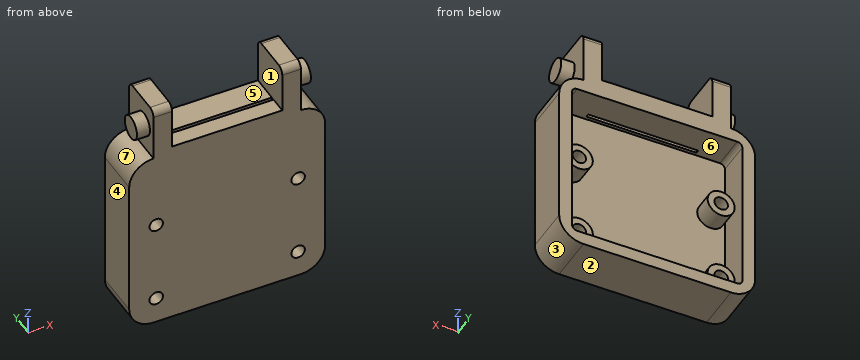
```python
from build123d import *

# Parameters (mm, degrees)
BOSS_EXTRUDE1_DEPTH   = 7
SKETCH2_R             = 2
CUT_EXTRUDE2_DEPTH    = 5
SKETCH3_R             = 2
CUT_EXTRUDE3_DEPTH    = 2
SKETCH4_W             = 16.3
SKETCH4_H             = 0.5
CUT_EXTRUDE4_DEPTH    = 2
F_2_0MM_DOWEL_HOLE1_D = 2
SKETCH8_W             = 21.826362025
SKETCH8_H             = 7
SKETCH8_W_2           = 16.3
SKETCH8_H_2           = 0.5
BOSS_EXTRUDE2_DEPTH   = 8
SKETCH9_R             = 1.75
BOSS_EXTRUDE3_DEPTH   = 2
LPATTERN4_COUNT       = 2
LPATTERN4_PITCH       = 23.75
SKETCH10_W            = 16.3
SKETCH10_H            = 7
CUT_EXTRUDE5_DEPTH    = 7
FILLET1_R             = 1


with BuildPart() as part:
    # Sketch1 → Boss-Extrude1 (new body)
    with BuildSketch(Plane(origin=(0, 0, 0), x_dir=(1, 0, 0), z_dir=(0, 1, 0))):
        with BuildLine():
            Line((-12.921525848, 14.392842997), (-12.921525848, -6.433519028))
            ThreePointArc((-12.921525848, -6.433519028), (-11.87097089, -8.969783057), (-9.334706861, -10.020338016))
            Line((-9.334706861, -10.020338016), (12.491655164, -10.020338016))
            ThreePointArc((12.491655164, -10.020338016), (15.027919193, -8.969783057), (16.078474152, -6.433519028))
            Line((16.078474152, -6.433519028), (16.078474152, 14.392842997))
            ThreePointArc((16.078474152, 14.392842997), (15.027919193, 16.929107026), (12.491655164, 17.979661984))
            Line((12.491655164, 17.979661984), (-9.334706861, 17.979661984))
            ThreePointArc((-9.334706861, 17.979661984), (-11.87097089, 16.929107026), (-12.921525848, 14.392842997))
        make_face()
    extrude(amount=BOSS_EXTRUDE1_DEPTH)

    # Sketch2 → Cut-Extrude2 (cut)
    with BuildSketch(Plane(origin=(0, 7, 0), x_dir=(1, 0, 0), z_dir=(0, 1, 0))):
        with BuildLine():
            Line((-10.27448552, 16.079661984), (13.431433823, 16.079661984))
            ThreePointArc((13.431433823, 16.079661984), (13.959671105, 15.860858938), (14.178474152, 15.332621656))
            Line((14.178474152, 15.332621656), (14.178474152, -7.373297687))
            ThreePointArc((14.178474152, -7.373297687), (13.959671105, -7.901534969), (13.431433823, -8.120338016))
            Line((13.431433823, -8.120338016), (-10.27448552, -8.120338016))
            ThreePointArc((-10.27448552, -8.120338016), (-10.802722802, -7.901534969), (-11.021525848, -7.373297687))
            Line((-11.021525848, -7.373297687), (-11.021525848, 15.332621656))
            ThreePointArc((-11.021525848, 15.332621656), (-10.802722802, 15.860858938), (-10.27448552, 16.079661984))
        make_face()
        with Locations((-8.921525848, 13.979661984)):
            Circle(SKETCH2_R, mode=Mode.SUBTRACT)
        with Locations((12.078474152, 13.979661984)):
            Circle(SKETCH2_R, mode=Mode.SUBTRACT)
        with Locations((-8.921525848, 1.479661984)):
            Circle(SKETCH2_R, mode=Mode.SUBTRACT)
        with Locations((12.078474152, 1.479661984)):
            Circle(SKETCH2_R, mode=Mode.SUBTRACT)
    extrude(amount=-CUT_EXTRUDE2_DEPTH, mode=Mode.SUBTRACT)

    # Sketch3 → Cut-Extrude3 (cut)
    with BuildSketch(Plane(origin=(0, 7, 0), x_dir=(1, 0, 0), z_dir=(0, 1, 0))):
        with Locations((12.078474152, 13.979661984)):
            Circle(SKETCH3_R)
        with Locations((12.078474152, 1.479661984)):
            Circle(SKETCH3_R)
        with Locations((-8.921525848, 13.979661984)):
            Circle(SKETCH3_R)
        with Locations((-8.921525848, 1.479661984)):
            Circle(SKETCH3_R)
    extrude(amount=-CUT_EXTRUDE3_DEPTH, mode=Mode.SUBTRACT)

    # Sketch4 → Cut-Extrude4 (cut)
    with BuildSketch(Plane.XY.offset(10.020338016)):
        with Locations((1.578474152, 2.75)):
            Rectangle(SKETCH4_W, SKETCH4_H)
    extrude(amount=-CUT_EXTRUDE4_DEPTH, mode=Mode.SUBTRACT)

    # Ø2.0mm Dowel Hole1 (through all)
    with Locations(Plane(origin=(0, 5, 0), x_dir=(1, 0, 0), z_dir=(0, 1, 0))):
        with Locations((12.078474152, 1.479661984), (12.078474152, 13.979661984), (-8.921525848, 1.479661984), (-8.921525848, 13.979661984)):
            Hole(F_2_0MM_DOWEL_HOLE1_D / 2)

    # Sketch8 → Boss-Extrude2 (add)
    with BuildSketch(Plane.XY.offset(10.020338016)):
        with Locations((1.578474152, 3.5)):
            Rectangle(SKETCH8_W, SKETCH8_H)
        with Locations((1.578474152, 2.75)):
            Rectangle(SKETCH8_W_2, SKETCH8_H_2, mode=Mode.SUBTRACT)
    extrude(amount=BOSS_EXTRUDE2_DEPTH)

    # Sketch9 → Boss-Extrude3 (add)
    with BuildSketch(Plane(origin=(12.491655164, 0, 0), x_dir=(0, 0, -1), z_dir=(1, 0, 0))):
        with Locations((-14.020338016, 2.75)):
            Circle(SKETCH9_R)
    boss_extrude3 = extrude(amount=BOSS_EXTRUDE3_DEPTH)

    # LPattern4: Boss-Extrude3 ×2
    with Locations(*[(-i * LPATTERN4_PITCH, 0, 0) for i in range(1, LPATTERN4_COUNT)]):
        add(boss_extrude3)

    # Sketch10 → Cut-Extrude5 (cut)
    with BuildSketch(Plane.XY.offset(18.020338016)):
        with Locations((1.578474152, 3.5)):
            Rectangle(SKETCH10_W, SKETCH10_H)
    extrude(amount=-CUT_EXTRUDE5_DEPTH, mode=Mode.SUBTRACT)

    # Fillet1
    fillet1_edges = [part.edges().sort_by_distance(p)[0] for p in [
        (-7.953116354, 0, 18.020338016),
        (11.110064658, 7, 18.020338016),
        (11.110064658, 0, 18.020338016),
        (-7.953116354, 7, 18.020338016),
    ]]
    fillet(fillet1_edges, radius=FILLET1_R)


solid = part.part
```
The listing builds one solid part. Answer for the finished solid, in the listing's coordinates (mm). Face numbers are marked on the shaded views. A direction names the side the tool comes from. Coordinates: 2 decimals unless noted, no trailing zeros. Loops run counter-clockwise (first coordinate to the right, second up) from the corner with the lowest first, then second, coordinate; pieces in that order, holes last. Notation, with made-up numbers: M 47.5,89 L 75.5,89 A18 cw 75.5,120 Z; hole C 47.5,72 d2. An arc over 180 degrees is marked long. Answer as a JSON object with one key per item and string values. Group by question number.
Item 1: Section B-B (z = 15) is taken. Write down the section's boundary in (x, y).
Item 2: Section D-D (z = 4) is taken. Write down the section's boundary in (x, y), and give its area (3 significant figures).
Item 3: Each of these flat-tipped pins is pushed along its axis until it touches: P1, Ø3, axis at x = -8.5, z = -2, coming from the +Y side; P2, Ø3, axis at y = 2, z = 13, coming from the +X side; P3, Ø1.5, axis at x = -4, y = 5, coming from the +Z side; P4, Ø3, axis at x = -8.92, z = -1.48, coming from the -Y side. Where does it stop, or does it pass through?
Item 4: Section C-C (z = 10.5) is taken. Write down the section's boundary in (x, y).
Item 5: Section A-A (x = -4.5) is taken. Write down the section's boundary in (y, z).
Item 6: Which of the six approach directions +Z, -Z, +X, -X, +Y, -Y give full straight-line access (tool end or side, diameter ignored) to the marked faces 4, 5, 6 and 7?
Item 7: Consider L1, parallel to X at y = 6.75, z = -9; L2, parallel to Z at x = 9.25, y = 4.5; L3, parallel to Z at x = -8.25, y = 1.75. Determine where each line is inside the solid, lowest interval first.
Item 8: Determine the mould class of the marked faces 1, 2 and 3 for opening direction X: +X half, -X half, draft (parallel to the pull), parting line (faces both ways), or undercut.
Solved:
{
 "1": {"outline": "M -11.26,1.3 L -9.33,1.3 L -9.33,0 L -6.57,0 L -6.57,7 L -9.33,7 L -9.33,4.2 L -11.26,4.2 Z; M 9.73,0 L 12.49,0 L 12.49,1.3 L 14.49,1.3 L 14.49,4.2 L 12.49,4.2 L 12.49,7 L 9.73,7 Z"},
 "2": {"outline": "M -12.92,0 L 16.08,0 L 16.08,7 L 14.18,7 L 14.18,2 L -11.02,2 L -11.02,7 L -12.92,7 Z", "area": "77.0 mm2"},
 "3": {"P1": "stops at y = 5", "P2": "stops at x = 14.49", "P3": "stops at z = 11.02", "P4": "stops at y = 0"},
 "4": {"outline": "M -9.33,0 L 12.49,0 L 12.49,7 L -9.33,7 Z; hole M -6.57,2.5 L 9.73,2.5 L 9.73,3 L -6.57,3 Z"},
 "5": {"outline": "M 0,-17.98 L 7,-17.98 L 7,-16.08 L 2,-16.08 L 2,8.12 L 2.5,8.12 L 2.5,11.02 L 0,11.02 Z; M 3,8.12 L 7,8.12 L 7,11.02 L 3,11.02 Z"},
 "6": {"face 4": "+Z, -Z, -X, +Y, -Y", "face 5": "+Z, +Y, -Y", "face 6": "+Y", "face 7": "-X, +Y, -Y"},
 "7": {"L1": "x = -12.92 to -11.02, 14.18 to 16.08", "L2": "z = -17.98 to -16.08, 8.12 to 11.02", "L3": "z = -17.98 to -14.72, -13.24 to -2.22, -0.74 to 18.02"},
 "8": {"face 1": "undercut", "face 2": "draft", "face 3": "+X half"}
}
